```python
from build123d import *

# Parameters (mm, degrees)
SKETCH2_W                = 35.36820513
SKETCH2_H                = 29.473504274
BOSS_EXTRUDE1_DEPTH      = 5.08
BOSS_EXTRUDE2_DEPTH      = 15.24
BOSS_EXTRUDE2_DEPTH_BACK = 15.24
SKETCH3_R                = 1.778


with BuildPart() as part:
    # Sketch2 → Boss-Extrude1 (new body)
    with BuildSketch(Plane(origin=(0, 0, 0), x_dir=(1, 0, 0), z_dir=(0, 1, 0))):
        with BuildLine():
            Line((-20.828, -15.875), (-20.828, 15.875))
            ThreePointArc((-20.828, 15.875), (-20.307235857, 17.132235857), (-19.05, 17.653))
            Line((-19.05, 17.653), (19.05, 17.653))
            ThreePointArc((19.05, 17.653), (20.307235857, 17.132235857), (20.828, 15.875))
            Line((20.828, 15.875), (20.828, -15.875))
            ThreePointArc((20.828, -15.875), (20.307235857, -17.132235857), (19.05, -17.653))
            Line((19.05, -17.653), (-19.05, -17.653))
            ThreePointArc((-19.05, -17.653), (-20.307235857, -17.132235857), (-20.828, -15.875))
        make_face()
        Rectangle(SKETCH2_W, SKETCH2_H, mode=Mode.SUBTRACT)
    extrude(amount=BOSS_EXTRUDE1_DEPTH)

    # Sketch3 → Boss-Extrude2 (add, two sides: drawn at the far end of the back side and taken through both)
    with BuildSketch(Plane(origin=(0, 5.08, 0), x_dir=(1, 0, 0), z_dir=(0, 1, 0)).offset(-BOSS_EXTRUDE2_DEPTH_BACK)):
        with Locations(Location((-19.05, -15.875, 0), (0, 0, 270))):
            Circle(SKETCH3_R)
        with Locations(Location((19.05, -15.875, 0), (0, 0, 270))):
            Circle(SKETCH3_R)
        with Locations(Location((19.05, 15.875, 0), (0, 0, 270))):
            Circle(SKETCH3_R)
        with Locations(Location((-19.05, 15.875, 0), (0, 0, 270))):
            Circle(SKETCH3_R)
    extrude(amount=BOSS_EXTRUDE2_DEPTH + BOSS_EXTRUDE2_DEPTH_BACK)


solid = part.part
```
Verification items for the finished model (mm, model axes). A direction names the side the tool comes from. Round coordinates to 2 decimals unless told otherwise and drop trailing zeros. Write each loop counter-clockwise with the first axis right and the second up, starting at its lowest first coordinate (ties: lowest second). Pieces come first, ordered by that corner, then holes. Notation, with made-up numbers: (-11.75, 35) - (28.25, 35) arc R19 cw to (28.25, 39) - close; hole circle Ø9 at (-37.75, -37.5). An arc over 180 degrees is marked (long way). Answer as a JSON object with one key per item and string values. Group by question number.
Q1. Section check B-B, the plane z = -5.5. Enter the section's corners in (x, y), plus the area to 3 significant figures.
Q2. Go/stop test with flat-tipped pins: pin 1 Ø0.9 at (x, z) = (-8, -16) entering from -Y; pin 2 Ø2.5 at (x, z) = (-7.5, 16.5) entering from +Y; pin 3 Ø5 at (y, z) = (-3.5, 12) entering from +X. Record where each tip stops, or that it passes through.
Q3. Thickness scan on line 1 (Z direction, x = -16.5, y = 5); line 2 (X direction, y = 4, z = -14); line 3 (X direction, y = -5, z = -15.5). Record the ranges inside material, lowest first.
Q4. Section check A-A, the plane x = -6.5. Enter the section's corners in (y, z), plus the area to 3 significant figures.
Q5. Section check C-C, the plane y = -2. Enter the section's corners in (x, z) (3 decimals).
Q6. Tool access check on faces 5 (the flat face through (17.684, 3, 0)), 6 (the flat face through (20.828, 3, 0)), 7 (the cylindrical face through (-20.786, 4.867, -16.26)). Record the directions out of +Z, -Z, +X, -X, +Y, -Y that give a thin tool (end or side, any length) a straight path to the whole face; none if there is none.
Q7. Mould release check, pull along Z, two halves, no side actions. Record for faces 1 (the flat face through (0, 3, 17.653)), 2 (the flat face through (19, -10.16, 16)), 3 (the cylindrical face through (20.55, 4.87, 16.83)), 4 (the flat face through (0, 3, 14.737)): released by +Z, released by -Z, zero draft, split by the parting line, or undercut.
Found:
{
 "1": {"outline": "(-20.83, 0) - (-17.68, 0) - (-17.68, 5.08) - (-20.83, 5.08) - close; (17.68, 0) - (20.83, 0) - (20.83, 5.08) - (17.68, 5.08) - close", "area": "31.9 mm^2"},
 "2": {"pin 1": "stops at y = 0", "pin 2": "stops at y = 5.08", "pin 3": "stops at x = 20.18"},
 "3": {"line 1": "z = -17.65 to -14.74, 14.74 to 17.65", "line 2": "x = -20.83 to -17.68, 17.68 to 20.83", "line 3": "x = -20.79 to -17.31, 17.31 to 20.79"},
 "4": {"outline": "(0, -17.65) - (5.08, -17.65) - (5.08, -14.74) - (0, -14.74) - close; (0, 14.74) - (5.08, 14.74) - (5.08, 17.65) - (0, 17.65) - close", "area": "29.6 mm^2"},
 "5": {"outline": "circle Ø3.556 at (-19.05, -15.875); circle Ø3.556 at (-19.05, 15.875); circle Ø3.556 at (19.05, -15.875); circle Ø3.556 at (19.05, 15.875)"},
 "6": {"face 5": "+Y, -Y", "face 6": "+Z, -Z, +X, +Y, -Y", "face 7": "none"},
 "7": {"face 1": "released by +Z", "face 2": "zero draft", "face 3": "undercut", "face 4": "undercut"}
}
